Job drawing, mm, ordinate dimensions from the low corner. One solid piece. A direction names the side the tool comes from. Round coordinates to 2 decimals unless told otherwise and drop trailing zeros. Loops run counter-clockwise (first coordinate to the right, second up) from the corner with the lowest first, then second, coordinate; pieces in that order, holes last.
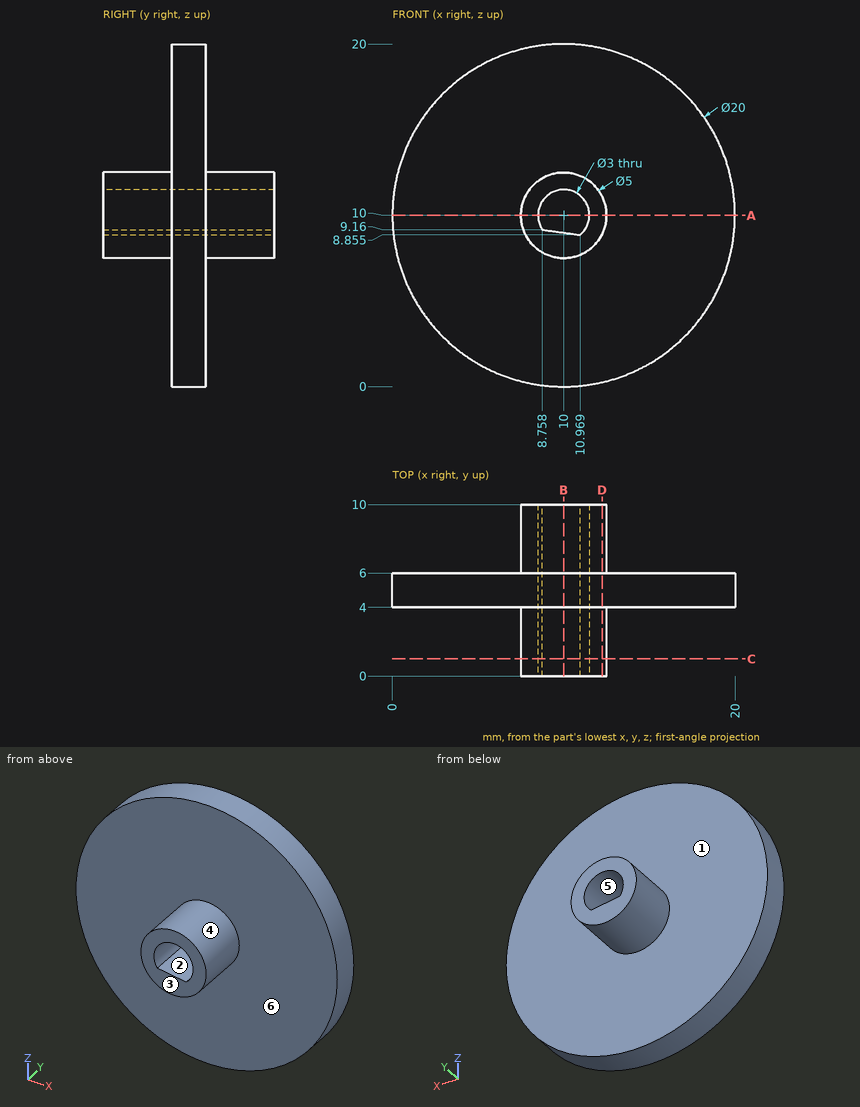
1) Slice it at C-C, the plane y = 1. Give the cut face in (x, z) (1 decimal).
Values:
outline: circle Ø5 at (10, 10); hole (8.8, 9.2) - (11, 8.9) arc R1.5 ccw (long way) to start
2) Wall check: line 1 along Y through (x, z) = (3, 5.25); line 2 along Z through (x, y) = (9.25, 9.5) (1 decimal); line 3 along X through (y, z) = (9.75, 8). Give the ranges that are in metal, low to high.
Values:
line 1: y = 4 to 6
line 2: z = 7.6 to 9.1, 11.3 to 12.4
line 3: x = 8.5 to 11.5
3) Slice it at A-A, the plane z = 10. Give the cut face in (x, y).
Values:
outline: (0, 4) - (7.5, 4) - (7.5, 0) - (8.5, 0) - (8.5, 10) - (7.5, 10) - (7.5, 6) - (0, 6) - close; (11.5, 0) - (12.5, 0) - (12.5, 4) - (20, 4) - (20, 6) - (12.5, 6) - (12.5, 10) - (11.5, 10) - close
4) Mould opens along Z. For the marked faces 4, 5 and 6 say: released by +Z, released by -Z, zero draft, split by the parting line, or undercut.
Values:
face 4: split by the parting line
face 5: undercut
face 6: zero draft
5) Tool access for the marked faces 1, 2 and 3: list every direction of +Z, -Z, +X, -X, +Y, -Y with a clear straight run to the whole face (end or side of a thin tool).
Values:
face 1: +Y
face 2: +Y, -Y
face 3: +Z, -Z, +X, -X, -Y
6) Drop flat-ended pins along their axis: pin 1 Ø1.5 at (x, y) = (12.5, 2.5) entering from -Z (1 decimal); pin 2 Ø1 at (y, z) = (4, 13) entering from -X; pin 3 Ø2 at (x, y) = (16.5, 5) entering from -Z. Give the stop position or say it passes through.
Values:
pin 1: stops at z = 8.2
pin 2: stops at x = 0.32
pin 3: stops at z = 1.65
7) Slice it at D-D, the plane x = 12.25. Give the cut face in (y, z).
Values:
outline: (0, 8.91) - (4, 8.91) - (4, 0.26) - (6, 0.26) - (6, 8.91) - (10, 8.91) - (10, 11.09) - (6, 11.09) - (6, 19.74) - (4, 19.74) - (4, 11.09) - (0, 11.09) - close
8) Slice it at B-B, the plane x = 10. Give the cut face in (y, z).
Values:
outline: (0, 7.5) - (4, 7.5) - (4, 0) - (6, 0) - (6, 7.5) - (10, 7.5) - (10, 8.99) - (0, 8.99) - close; (0, 11.5) - (10, 11.5) - (10, 12.5) - (6, 12.5) - (6, 20) - (4, 20) - (4, 12.5) - (0, 12.5) - close
